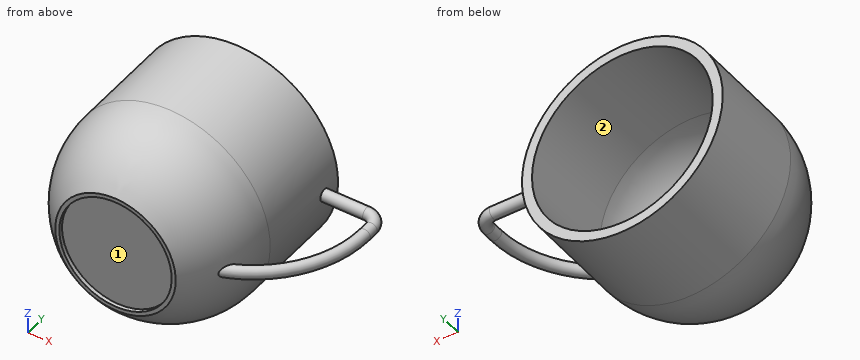
```python
from build123d import *

# Parameters (mm, degrees)
SKETCH11_R         = 3
SKETCH14_R         = 28
CUT_EXTRUDE1_DEPTH = 2


# Read off the part's stored shape, not the designer's step: Shell4
with BuildPart() as part:
    # Sketch2 → Revolve1 (revolve)
    with BuildSketch(Plane.XY, mode=Mode.PRIVATE) as revolve1_sk:
        with BuildLine():
            Line((-40.101497772, 45), (-40.101497772, -45))
            Line((-40.101497772, -45), (-10.101497772, -45))
            ThreePointArc((-10.101497772, -45), (4.619861778, -27.360679775), (9.898502228, -5))
            Line((9.898502228, -5), (9.898502228, 45))
            Line((9.898502228, 45), (-40.101497772, 45))
        make_face()
    revolve(revolve1_sk.sketch.rotate(Axis((-40.101497772, 45, 0), (0, -1, 0)), 90), axis=Axis((-40.101497772, 45, 0), (0, -1, 0)))

    # Sweep16: sweep along a path in Sketch3
    with BuildLine(Plane.XY) as sweep16_path:
        Line((7.898502228, 35), (30.898502228, 35))
        ThreePointArc((30.898502228, 35), (35.848249696, 32.949747468), (37.898502228, 28))
        Line((37.898502228, 28), (37.898502228, 23))
        ThreePointArc((37.898502228, 23), (27.703635862, -8.898275815), (0.898502228, -28.971145841))
    # Sketch11 → Sweep16 (sweep)
    with BuildSketch(Plane(origin=(7.898502228, 0, 0), x_dir=(0, 0, -1), z_dir=(1, 0, 0))):
        with Locations((0, 35)):
            Circle(SKETCH11_R)
    sweep(path=sweep16_path.line)

    # Sketch14 → Cut-Extrude1 (cut)
    with BuildSketch(Plane.XZ.offset(45)):
        with Locations(Location((-40.101497772, 0, 0), (0, 0, 270))):
            Circle(SKETCH14_R)
    extrude(amount=-CUT_EXTRUDE1_DEPTH, mode=Mode.SUBTRACT)

    # Shell4 outline → Shell4 (revolve, cut)
    with BuildSketch(Plane(origin=(-40.101497772, 0, 0), x_dir=(1, 0, 0), z_dir=(0, 0, 1))):
        with BuildLine():
            ThreePointArc((32.999999984, -35.594117098), (41.89272013, -21.431676729), (45, -4.999999985))
            Line((45, -4.999999985), (45, 45))
            Line((45, 45), (0, 45))
            Line((0, 45), (0, -35))
            Line((0, -35), (33, -35))
            Line((33, -35), (32.999999984, -35.594117098))
        make_face()
    revolve(axis=Axis((-40.101497772, 0, 0), (0, 1, 0)), mode=Mode.SUBTRACT)


solid = part.part
```
For this review, take the finished solid that the model builds, in its own axes (mm). Face numbers are marked on the shaded views. Coordinates: 2 decimals unless noted, no trailing zeros. Write each loop counter-clockwise with the first axis right and the second up, starting at its lowest first coordinate (ties: lowest second). Pieces come first, ordered by that corner, then holes.
(1) For pin 1 Ø8 at (x, y) = (-5.5, -23) entering from +Z; pin 2 Ø10 at (x, y) = (-30, 33) entering from -Z; pin 3 Ø1.5 at (y, z) = (-16.5, 8) entering from -X, all flat-tipped, find the tip position at first contact; note any pin that passes through.
(2) Add section A-A on z = 0. Give the boundary of the cut face in (x, y).
(3) The part is to be moulded in two halves that separate along X. For the marked faces 1 and 2, say which applies: +X half, -X half, draft (parallel to the pull), parting line (faces both ways), or undercut.
(4) Add section B-B on z = 36. Give the boundary of the cut face in (x, y), then the cut area to 3 significant figures.
(5) Add section C-C on x = 0. Give the boundary of the cut face in (y, z), then the cut area to 3 significant figures.
(6) Add section D-D on y = 3. Count the separate pieces of the cut face and the enclosed holes in it, then the cut area to 3 significant figures.
(7) Wall thickness on probe 1 along X at (y, z) = (23, 0); probe 2 along X at (y, z) = (11, 0); probe 3 along X at (y, z) = (-43.9, 0): over which ranges is each line inside the solid? List them lowest first.
Answer sheet:
1. pin 1: stops at z = 35.7
1. pin 2: stops at z = -49.74
1. pin 3: stops at x = -88.31
2. outline: (-90.1, -5) arc R50 ccw to (-70.1, -45) - (-68.1, -45) - (-68.1, -43) - (-12.1, -43) - (-12.1, -45) - (-10.1, -45) arc R50 ccw to (2.17, -31.7) arc R58 ccw to (40.9, 23) - (40.9, 28) arc R10 ccw to (30.9, 38) - (9.9, 38) - (9.9, 45) - (4.9, 45) - (4.9, -5) arc R45 cw to (-7.1, -35.59) - (-7.1, -35) - (-73.1, -35) - (-73.1, -35.59) arc R45 cw to (-85.1, -5) - (-85.1, 45) - (-90.1, 45) - close; hole (6.39, -23.39) arc R52 ccw to (34.9, 23) - (34.9, 28) arc R4 ccw to (30.9, 32) - (9.9, 32) - (9.9, -5) arc R50 cw to start
3. face 1: undercut
3. face 2: undercut
4. outline: (-74.8, -5) arc R34.7 ccw to (-5.4, -5) - (-5.4, 45) - (-13.1, 45) - (-13.1, -5) arc R27 cw to (-67.1, -5) - (-67.1, 45) - (-74.8, 45) - close
4. area: 1,520 mm2
5. outline: (-5, -29.86) - (45, -29.86) - (45, -20.42) - (-5, -20.42) arc R20.42 cw to (-5, 20.42) - (45, 20.42) - (45, 29.86) - (-5, 29.86) arc R29.86 ccw to start
5. area: 1,690 mm2
6. separate pieces: 2
6. enclosed holes: 1
6. area: 1,520 mm2
7. probe 1: x = -90.1 to -85.1, 4.9 to 9.9, 34.9 to 40.9
7. probe 2: x = -90.1 to -85.1, 4.9 to 9.9, 33.49 to 39.64
7. probe 3: x = -71.51 to -68.1, -12.1 to -8.69
